```python
from build123d import *

# Parameters (mm, degrees)
SKETCH1_W           = 20
SKETCH1_H           = 41
SKETCH1_W_2         = 6
SKETCH1_H_2         = 25
SKETCH1_R           = 1.75
BOSS_EXTRUDE1_DEPTH = 4
SKETCH1_3_W         = 6
SKETCH1_3_H         = 25
SKETCH1_3_H_2       = 12.5
BOSS_EXTRUDE2_DEPTH = 29
SKETCH2_R           = 9.55
CUT_EXTRUDE1_DEPTH  = 29
RIB1_REACH          = 50.27
SKETCH3_WALL_W      = 112.866695872
SKETCH3_WALL_H      = 2.95
RIB7_REACH          = 50.27
SKETCH4_WALL_W      = 112.866695872
SKETCH4_WALL_H      = 2.95
CUT_EXTRUDE4_START  = 1.5
SKETCH1_4_R         = 1.75
CUT_EXTRUDE4_DEPTH  = 2.5
SKETCH5_W           = 25
SKETCH5_H           = 25
SKETCH5_R           = 3.05
BOSS_EXTRUDE3_DEPTH = 2
SKETCH6_R           = 9.55
CUT_EXTRUDE5_DEPTH  = 0.2


with BuildPart() as part:
    # Sketch1 → Boss-Extrude1 (new body)
    with BuildSketch(Plane(origin=(0, 0, 0), x_dir=(1, 0, 0), z_dir=(0, 1, 0))):
        with Locations((10, 12.5)):
            Rectangle(SKETCH1_W, SKETCH1_H)
        with Locations((10, 12.5)):
            Rectangle(SKETCH1_W_2, SKETCH1_H_2, mode=Mode.SUBTRACT)
        with Locations(Location((4, -4, 0), (0, 0, 270))):
            Circle(SKETCH1_R, mode=Mode.SUBTRACT)
        with Locations(Location((4, 29, 0), (0, 0, 270))):
            Circle(SKETCH1_R, mode=Mode.SUBTRACT)
        with Locations(Location((16, -4, 0), (0, 0, 270))):
            Circle(SKETCH1_R, mode=Mode.SUBTRACT)
        with Locations(Location((16, 29, 0), (0, 0, 270))):
            Circle(SKETCH1_R, mode=Mode.SUBTRACT)
    extrude(amount=BOSS_EXTRUDE1_DEPTH)

    # Sketch1<3> → Boss-Extrude2 (add)
    with BuildSketch(Plane(origin=(0, 0, 0), x_dir=(1, 0, 0), z_dir=(0, 1, 0))):
        with Locations((10, 12.5)):
            Rectangle(SKETCH1_3_W, SKETCH1_3_H)
        with Locations((10, 18.75)):
            Rectangle(SKETCH1_3_W, SKETCH1_3_H_2)
    extrude(amount=BOSS_EXTRUDE2_DEPTH)

    # Sketch2 → Cut-Extrude1 (cut)
    with BuildSketch(Plane(origin=(13, 0, 0), x_dir=(0, 0, -1), z_dir=(1, 0, 0))):
        with Locations((12.5, 16.5)):
            Circle(SKETCH2_R)
    extrude(amount=-CUT_EXTRUDE1_DEPTH, mode=Mode.SUBTRACT)

    # Sketch3 wall → Rib1 (add, up to next)
    with BuildSketch(Plane(origin=(16.5, 10.25, 0), x_dir=(0.488603368932, -0.87250601595, 0), z_dir=(0.87250601595, 0.488603368932, 0)), mode=Mode.PRIVATE) as rib1_sk1:
        with Locations((0, 1.475)):
            Rectangle(SKETCH3_WALL_W, SKETCH3_WALL_H)
    rib1_tool1 = extrude(rib1_sk1.sketch, amount=-RIB1_REACH, mode=Mode.PRIVATE) - part.part
    rib1 = rib1_tool1.solids().sort_by_distance((16.5, 10.25, 0))[0]
    add(rib1)

    # Sketch4 wall → Rib7 (add, up to next)
    with BuildSketch(Plane(origin=(3.5, 10.25, 0), x_dir=(-0.488603368932, -0.87250601595, 0), z_dir=(0.87250601595, -0.488603368932, 0)), mode=Mode.PRIVATE) as rib7_sk1:
        with Locations((0, 1.475)):
            Rectangle(SKETCH4_WALL_W, SKETCH4_WALL_H)
    rib7_tool1 = extrude(rib7_sk1.sketch, amount=RIB7_REACH, mode=Mode.PRIVATE) - part.part
    rib7 = rib7_tool1.solids().sort_by_distance((3.5, 10.25, 0))[0]
    add(rib7)

    # Mirror1: Rib1, Rib7 across plane
    add(rib1.mirror(Plane.XY.offset(-12.5)))
    add(rib7.mirror(Plane.XY.offset(-12.5)))

    # Sketch1<4> → Cut-Extrude4 (cut)
    # profile 1 of 4: a face of its own
    with BuildSketch(Plane(origin=(0, 0, 0), x_dir=(1, 0, 0), z_dir=(0, 1, 0)).offset(CUT_EXTRUDE4_START)):
        Polygon((4, -0.709103466), (6.85, -2.354551733), (6.85, -5.645448267), (4, -7.290896534), (1.15, -5.645448267), (1.15, -2.354551733), align=None)
        with Locations(Location((4, -4, 0), (0, 0, 270))):
            Circle(SKETCH1_4_R, mode=Mode.SUBTRACT)
    # profile 2 of 4: a face of its own
    with BuildSketch(Plane(origin=(0, 0, 0), x_dir=(1, 0, 0), z_dir=(0, 1, 0)).offset(CUT_EXTRUDE4_START)):
        Polygon((1.15, 30.645448267), (1.15, 27.354551733), (4, 25.709103466), (6.85, 27.354551733), (6.85, 30.645448267), (4, 32.290896534), align=None)
        with Locations(Location((4, 29, 0), (0, 0, 270))):
            Circle(SKETCH1_4_R, mode=Mode.SUBTRACT)
    # profile 3 of 4: a face of its own
    with BuildSketch(Plane(origin=(0, 0, 0), x_dir=(1, 0, 0), z_dir=(0, 1, 0)).offset(CUT_EXTRUDE4_START)):
        Polygon((16, 25.709103466), (13.15, 27.354551733), (13.15, 30.645448267), (16, 32.290896534), (18.85, 30.645448267), (18.85, 27.354551733), align=None)
        with Locations(Location((16, 29, 0), (0, 0, 270))):
            Circle(SKETCH1_4_R, mode=Mode.SUBTRACT)
    # profile 4 of 4: a face of its own
    with BuildSketch(Plane(origin=(0, 0, 0), x_dir=(1, 0, 0), z_dir=(0, 1, 0)).offset(CUT_EXTRUDE4_START)):
        Polygon((18.85, -5.645448267), (18.85, -2.354551733), (16, -0.709103466), (13.15, -2.354551733), (13.15, -5.645448267), (16, -7.290896534), align=None)
        with Locations(Location((16, -4, 0), (0, 0, 270))):
            Circle(SKETCH1_4_R, mode=Mode.SUBTRACT)
    extrude(amount=CUT_EXTRUDE4_DEPTH, mode=Mode.SUBTRACT)

    # Sketch5 → Boss-Extrude3 (add)
    with BuildSketch(Plane.ZY.offset(-7)):
        with Locations((-12.5, 16.5)):
            Rectangle(SKETCH5_W, SKETCH5_H)
        with Locations((-12.5, 16.5)):
            Circle(SKETCH5_R, mode=Mode.SUBTRACT)
    extrude(amount=BOSS_EXTRUDE3_DEPTH)

    # SurfaceCut1
    split(bisect_by=Plane(origin=(10, 0, 0), x_dir=(0, 0, -1), z_dir=(1, 0, 0)), keep=Keep.BOTTOM)

    # Sketch6 → Cut-Extrude5 (cut)
    with BuildSketch(Plane(origin=(7, 0, 0), x_dir=(0, 0, -1), z_dir=(1, 0, 0))):
        with Locations((12.5, 16.5)):
            Circle(SKETCH6_R)
    extrude(amount=-CUT_EXTRUDE5_DEPTH, mode=Mode.SUBTRACT)


solid = part.part
```
Input: part model. Units: mm. Frame: model coordinates. A direction names the side the tool comes from. Round coordinates to 2 decimals unless told otherwise and drop trailing zeros. Loops run counter-clockwise (first coordinate to the right, second up) from the corner with the lowest first, then second, coordinate; pieces in that order, holes last. Notation, with made-up numbers: (80, 45.25) -> (120, 45.25) arc R25 ccw to (120, 65.25) -> close; hole circle Ø8 at (20, -9.75). An arc over 180 degrees is marked (long way). Write each question's results on one line, items separated by ' | '.
1. Mould query, pull axis Y, two halves, no side actions, for faces 6 (the face through (6.8, 19, -10)), 7 (the face through (2.7, 1.5, -27.6)), 8 (the face through (1.15, 3, -29)). Classes: +Y half, -Y half, draft (parallel to the pull), parting line (faces both ways), or undercut.
Geometry results:
face 6: undercut | face 7: +Y half | face 8: draft
2. Section C-C (x = 9). Return loops of the section in (y, z).
Geometry results:
outline: (0, -33) -> (4, -33) -> (4, -25) -> (29, -25) -> (29, 0) -> (4, 0) -> (4, 8) -> (0, 8) -> close; hole circle Ø19.1 at (16.5, -12.5)
3. Set-up query: faces 1 (the face through (7, 4, 4)), 2 (the face through (2.535, 8.527, -1.496)), 3 (the face through (2.56, 2.73, 1.54)), 4 (the face through (7, 4, -29)), 5 (the face through (2, 4, -13)). Return all of +Z, -Z, +X, -X, +Y, -Y with unobstructed straight access to the full face (end or side cutting, diameter ignored); none if empty.
Geometry results:
face 1: +Z, +X, -X, +Y | face 2: +Z, -Z, -X, +Y | face 3: +Y | face 4: -Z, +X, -X, +Y | face 5: -X, +Y
4. Ray query, line 1 (Y direction, x = 6.05, z = -12.5); line 2 (Z direction, x = 6, y = 16.5); line 3 (Y direction, x = 7.95, z = -12.5). Return the intervals inside material, ascending. Write a range as from..to.
Geometry results:
line 1: 0..13.45, 19.55..29 | line 2: -25..-15.55, -9.45..0 | line 3: 0..6.95, 26.05..29
5. Section B-B (z = -29). Return loops of the section in (x, y), and give its area (3 significant figures).
Geometry results:
outline: (0, 0) -> (2.25, 0) -> (2.25, 1.5) -> (1.15, 1.5) -> (1.15, 4) -> (0, 4) -> close; (5.75, 0) -> (10, 0) -> (10, 4) -> (6.85, 4) -> (6.85, 1.5) -> (5.75, 1.5) -> close | area: 20.5 mm2
6. First-contact query: P1, Ø1, axis at x = 6, z = 4, coming from the +Y side; P2, Ø2.5, axis at x = 1.5, y = 7, coming from the -Z side; P3, Ø2, axis at y = 21, z = -13, coming from the -X side. Flat tips, straight axial feed; report the tip coordinate or a pass-through.
Geometry results:
P1: y = 1.5 | P2: z = -25 | P3: x = 5
7. Section D-D (x = 3.25). Return loops of the section in (y, z), and give its area (3 significant figures).
Geometry results:
outline: (0, -33) -> (4, -33) -> (4, -31.86) -> (1.5, -31.86) -> (1.5, -30.58) -> (0, -30.58) -> close; (0, -27.42) -> (1.5, -27.42) -> (1.5, -26.14) -> (4, -26.14) -> (4, -25) -> (9.8, -25) -> (9.8, -22.05) -> (4, -22.05) -> (4, -2.95) -> (9.8, -2.95) -> (9.8, 0) -> (4, 0) -> (4, 1.14) -> (1.5, 1.14) -> (1.5, 2.42) -> (0, 2.42) -> close; (0, 5.58) -> (1.5, 5.58) -> (1.5, 6.86) -> (4, 6.86) -> (4, 8) -> (0, 8) -> close | area: 160 mm2
8. Section A-A (y = 16.5). Return loops of the section in (x, z).
Geometry results:
outline: (5, -25) -> (10, -25) -> (10, -22.05) -> (6.8, -22.05) -> (6.8, -15.55) -> (5, -15.55) -> close; (5, -9.45) -> (6.8, -9.45) -> (6.8, -2.95) -> (10, -2.95) -> (10, 0) -> (5, 0) -> close
